Source: three-view drawing plus pictorial views. Frame: mm from the lowest corner of the part. Coordinates: 2 decimals unless noted, no trailing zeros. Write each loop counter-clockwise with the first axis right and the second up, starting at its lowest first coordinate (ties: lowest second). Pieces come first, ordered by that corner, then holes. Notation, with made-up numbers: (-20.5, -31) - (-12.5, -31) arc R24 cw to (-12.5, 1) - close; hole circle Ø1 at (-39.5, 72). An arc over 180 degrees is marked (long way). Put each result on its own line as item: value. Start each with the question number.
1. Pull-direction query (X, two-part tool) for the marked faces 1, 2 and 3; classes: released by +X, released by -X, zero draft, split by the parting line, or undercut.
2. Cut plane D-D, the plane x = 29.5. Return loops of the section in (y, z) (1 decimal), and give its area (3 significant figures).
3. Cut plane A-A, the plane y = 35. Return loops of the section in (x, z).
4. Cut plane B-B, the plane x = 22.5. Return loops of the section in (y, z).
5. Pin query (flat end, axial travel): pin 1 (4.5 mm diameter, centred on x = 49.2, y = 40.48, fed in from +Z); pin 2 (1.5 mm diameter, centred on x = 48.5, z = 2.5, fed in from +Y); pin 3 (1.5 mm diameter, centred on y = 39, z = 12, fed in from -X); pin 4 (6 mm diameter, centred on y = 44.5, z = 3.5, fed in from -X). Return the tip coordinate at first contact, or that it passes through.
6. Cut plane C-C, the plane z = 8.5. Count the separate pieces of the cut face and the enclosed holes in it, and give its area (3 significant figures).
7. Line query: line 1 (Y direction, x = 49.5, z = 10.25) (1 decimal); line 2 (X direction, y = 18, z = 3.5) (1 decimal); line 3 (Y direction, x = 9, z = 3.5). Output: solid intervals per line, ascending.
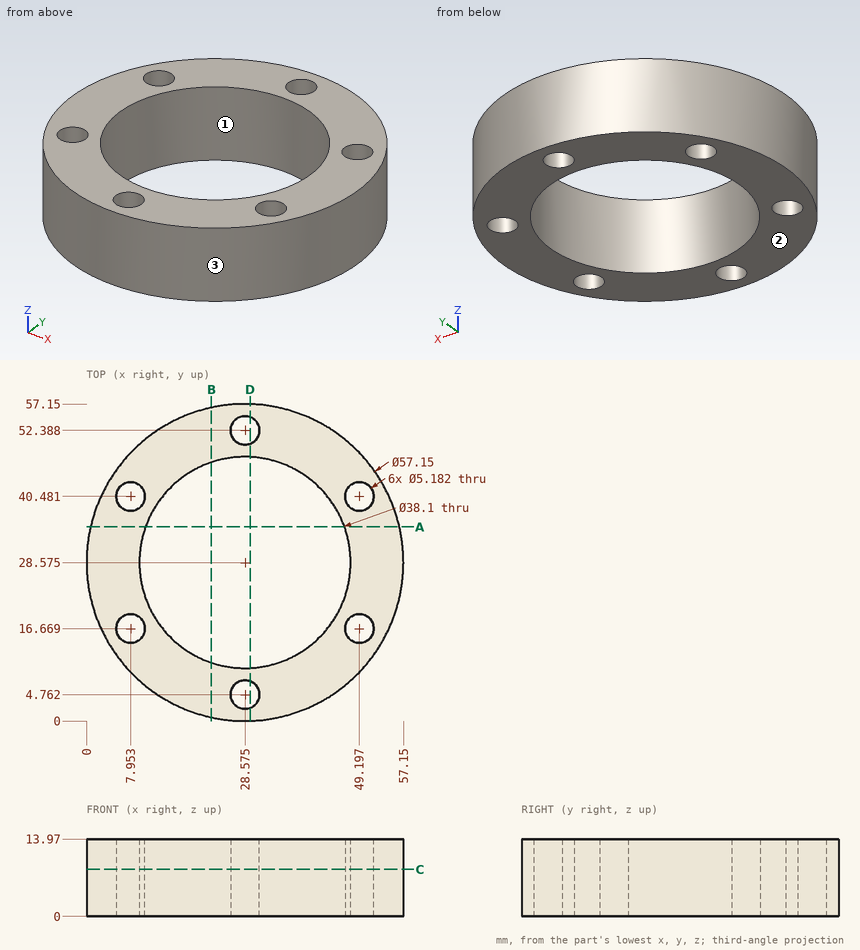
Report:
1. face 1: undercut
1. face 2: zero draft
1. face 3: split by the parting line
2. outline: (0, 0) - (2.3, 0) - (2.3, 14) - (0, 14) - close; (7.2, 0) - (9.5, 0) - (9.5, 14) - (7.2, 14) - close; (47.6, 0) - (50, 0) - (50, 14) - (47.6, 14) - close; (54.8, 0) - (57.1, 0) - (57.1, 14) - (54.8, 14) - close
2. area: 131 mm^2
3. outline: (0.73, 0) - (10.64, 0) - (10.64, 13.97) - (0.73, 13.97) - close; (46.51, 0) - (56.42, 0) - (56.42, 13.97) - (46.51, 13.97) - close
4. outline: (0.65, 0) - (10.52, 0) - (10.52, 13.97) - (0.65, 13.97) - close; (46.63, 0) - (56.5, 0) - (56.5, 13.97) - (46.63, 13.97) - close
5. pin 1: passes through
5. pin 2: stops at y = 49.76
5. pin 3: stops at x = 1.69
5. pin 4: stops at x = 3.09
6. separate pieces: 1
6. enclosed holes: 7
6. area: 1,300 mm^2
7. line 1: y = 9.1 to 14.1, 19.2 to 37.9, 43.1 to 48
7. line 2: x = 2 to 5.7, 10.2 to 12.7, 44.4 to 47, 51.4 to 55.1
7. line 3: y = 7.76 to 14.3, 19.04 to 38.11, 42.85 to 49.39
